Can you work these out from the model? Positions are in its coordinate system, mm. A direction names the side the tool comes from. Round coordinates to 2 decimals unless told otherwise and drop trailing zeros. Loops run counter-clockwise (first coordinate to the right, second up) from the corner with the lowest first, then second, coordinate; pieces in that order, holes last. Notation, with made-up numbers: (-10, -9) -> (23, -9) arc R35 ccw to (23, 30) -> close; hole circle Ø5 at (-25, -38). An arc over 180 degrees is marked (long way). Write each question's results on one line, items separated by ' | '.
from build123d import *

# Parameters (mm, degrees)
BOSS_EXTRUDE1_DEPTH             = 50.8
F_9_32_0_28125_DIAMETER_HOLE1_D = 7.14375


with BuildPart() as part:
    # Sketch1 → Boss-Extrude1 (new body)
    with BuildSketch(Plane.XY):
        with BuildLine():
            ThreePointArc((0.076969069, 5.862862723), (-1.78290287, 1.372734663), (-6.273030931, -0.487137277))
            Line((-6.273030931, -0.487137277), (6.426969069, -0.487137277))
            Line((6.426969069, -0.487137277), (19.126969069, -13.187137277))
            Line((19.126969069, -13.187137277), (31.826969069, -13.187137277))
            Line((31.826969069, -13.187137277), (31.826969069, 5.862862723))
            Line((31.826969069, 5.862862723), (12.908151542, 24.781680251))
            Line((12.908151542, 24.781680251), (-6.273030931, 24.781680251))
            Line((-6.273030931, 24.781680251), (-6.273030931, 12.212862723))
            ThreePointArc((-6.273030931, 12.212862723), (-1.78290287, 10.352990784), (0.076969069, 5.862862723))
        make_face()
        with BuildLine():
            ThreePointArc((-6.273030931, 12.212862723), (-12.623030931, 5.862862723), (-6.273030931, -0.487137277))
            Line((-6.273030931, -0.487137277), (-6.273030931, 12.212862723))
        make_face()
        with BuildLine():
            Line((-6.273030931, 12.212862723), (-6.273030931, -0.487137277))
            ThreePointArc((-6.273030931, -0.487137277), (-1.78290287, 1.372734663), (0.076969069, 5.862862723))
            ThreePointArc((0.076969069, 5.862862723), (-1.78290287, 10.352990784), (-6.273030931, 12.212862723))
        make_face()
    extrude(amount=-BOSS_EXTRUDE1_DEPTH)

    # 9/32 (0.28125) Diameter Hole1 (through all)
    with Locations(Plane(origin=(-6.273030931, 5.862862723, 0), x_dir=(1, 0, 0), z_dir=(0, 0, 1))):
        with Locations((0, 0)):
            Hole(F_9_32_0_28125_DIAMETER_HOLE1_D / 2)


solid = part.part
1. If we section it at B-B (x = -5): List the corners of the cut face in (y, z) for me.
Final values:
outline: (-0.49, -50.8) -> (2.53, -50.8) -> (2.53, 0) -> (-0.49, 0) -> close; (9.2, -50.8) -> (24.78, -50.8) -> (24.78, 0) -> (9.2, 0) -> close
2. If we section it at D-D (x = 3): List the corners of the cut face in (y, z) for me, then the cut area to 3 significant figures.
Final values:
outline: (-0.49, -50.8) -> (24.78, -50.8) -> (24.78, 0) -> (-0.49, 0) -> close | area: 1,280 mm2
3. If we section it at A-A (z = -37.5): List the corners of the cut face in (x, y) for me, then the cut area to 3 significant figures.
Final values:
outline: (-6.27, -0.49) -> (6.43, -0.49) -> (19.13, -13.19) -> (31.83, -13.19) -> (31.83, 5.86) -> (12.91, 24.78) -> (-6.27, 24.78) -> (-6.27, 12.21) arc R6.35 ccw to start; hole circle Ø7.14 at (-6.27, 5.86) | area: 1,050 mm2
4. On a 3-axis mill with a long thin cutter (end or side, diameter ignored), from which of +Z, -Z, +X, -X, +Y, -Y can I reach the whole of each face in a straight line? I mean faces 5 (the face through (-6.273, 19, -25)), 6 (the face through (-12.62, 6, -25.04)). Say none if no direction works.
Final values:
face 5: +Z, -Z, -X, +Y | face 6: +Z, -Z, -X
5. We'd pull the mould along Y, two halves only. Please class faces 1 (the face through (9, 6, -50.8)), 2 (the face through (-5.808, 9.404, -25.756)), 3 (the face through (3, 24.782, -25)), 4 (the face through (0, -0.487, -25)): pulls with the +Y half, pulls with the -Y half, needs draft (parallel to the pull), parting line crosses it, or undercut.
Final values:
face 1: needs draft | face 2: undercut | face 3: pulls with the +Y half | face 4: pulls with the -Y half
6. Please list where these lines run through material, in increasing order: line 1 (Y direction, x = -6.5, z = -41); line 2 (X direction, y = 6, z = -46); line 3 (X direction, y = 3, z = -31). Write a range as from..to.
Final values:
line 1: -0.48..2.3, 9.43..12.21 | line 2: -12.62..-9.84, -2.7..31.69 | line 3: -11.94..-8.41, -4.14..31.83
7. Will these pins go through, and if not, where does the flat tip stop? pin 1 (3 mm diameter, centred on x = 21, z = -37.5, fed in from +Y); pin 2 (14 mm diameter, centred on x = -2.5, z = -31, fed in from -Y); pin 3 (4 mm diameter, centred on y = 3.5, z = -35.5, fed in from -X).
Final values:
pin 1: y = 18.19 | pin 2: y = -0.49 | pin 3: x = -12.61
8. If we section it at C-C (y = 8.5): List the corners of the cut face in (x, z) for me.
Final values:
outline: (-12.05, -50.8) -> (-8.68, -50.8) -> (-8.68, 0) -> (-12.05, 0) -> close; (-3.86, -50.8) -> (29.19, -50.8) -> (29.19, 0) -> (-3.86, 0) -> close
